Build history of the part. All positions in model axes, mm. Face numbers are marked on the shaded views. Give positions to 0.01 mm unless a question says otherwise; leave off trailing zeros. Order: outer loops, then holes, each group sorted by start corner. A loop starts at its lowest first (then second) coordinate and runs counter-clockwise, first axis right, second up. Notation, with made-up numbers: (85, 78) - (137, 78) arc R24 ccw to (137, 97) - close; hole circle Ø2 at (30, 24). An arc over 180 degrees is marked (long way). Use a Markdown table: item, result. Add a question column.
(1) Slice it at A-A (y = 0). Write the cut outline in (x, z).
(2) Mould opens along X. For the marked faces 1, 2, 3 and 4 say: +X half, -X half, draft (parallel to the pull), parting line (faces both ways), or undercut.
(3) Wall check: line 1 (Y direction, x = 0, z = 5.5); line 2 (Y direction, x = 7.25, z = 1.5); line 3 (X direction, y = -1, z = 6). Give the ranges that are in metal, low to high.
(4) Slice it at C-C (z = 2.25). Write the cut outline in (x, y), then the cut area to 3 significant figures.
(5) Flat gauge pins, fed straight in: pin 1 (5 mm diameter, centred on x = -8.5, z = -1.5, fed in from +Y); pin 2 (16 mm diameter, centred on x = 0, y = 0, fed in from +Z); pin 3 (5 mm diameter, centred on y = 5.5, z = 5, fed in from +X). Where does each tip first touch, or does it go through?
Solid Edge part; units mm, degrees
sketch "Sketch1" plane through (0, 0, 0) normal (0, 0, 1) x (1, 0, 0)
  circle A0 centre (0, 0) radius 10.1
  circle A1 centre (0, 0) radius 14
extrude "Protrusion1" add sketch "Sketch1" along normal blind 12
sketch "Sketch2" plane through (0, 0, 0) normal (0, 0, -1) x (1, 0, 0)
  circle A0 centre (0, 0) radius 14
extrude "ExtrudedProtrusion_2" add sketch "Sketch2" along normal blind 4
sketch "Sketch3" plane through (0, 0, 0) normal (0, 0, 1) x (1, 0, 0)
  circle A0 centre (0, 0) radius 7
extrude "Cutout1" cut sketch "Sketch3" against normal through all
chamfer "Chamfer_1" distance 1 angle 45 1 edges at (-10.1, 0, 12)
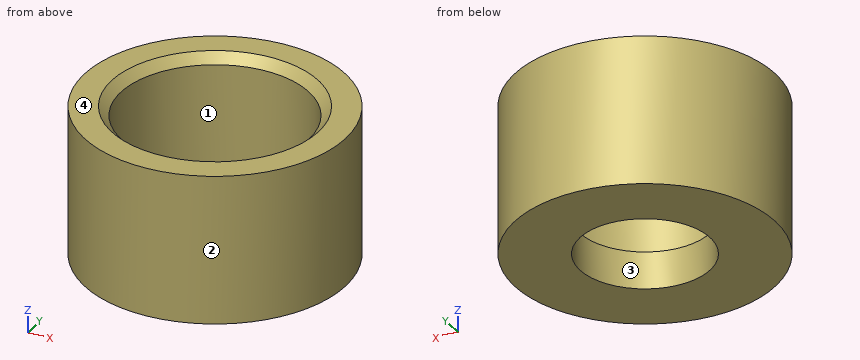
Solution:
| question | item | result |
|---|---|---|
| 1 | outline | (-14, -4) - (-7, -4) - (-7, 0) - (-10.1, 0) - (-10.1, 11) - (-11.1, 12) - (-14, 12) - close; (7, -4) - (14, -4) - (14, 12) - (11.1, 12) - (10.1, 11) - (10.1, 0) - (7, 0) - close |
| 2 | face 1 | undercut |
| 2 | face 2 | parting line |
| 2 | face 3 | undercut |
| 2 | face 4 | draft |
| 3 | line 1 | -14 to -10.1, 10.1 to 14 |
| 3 | line 2 | -11.98 to -7.03, 7.03 to 11.98 |
| 3 | line 3 | -13.96 to -10.05, 10.05 to 13.96 |
| 4 | outline | circle Ø28 at (0, 0); hole circle Ø20.2 at (0, 0) |
| 4 | area | 295 mm2 |
| 5 | pin 1 | y = 12.65 |
| 5 | pin 2 | z = 0 |
| 5 | pin 3 | x = 13.67 |
